from build123d import *

# Parameters (mm, degrees)
F1_DEPTH = 63.5
F2_DEPTH = 25.4
F0_W     = 25.4
F0_H     = 19.05
F3_DEPTH = 25.4
F4_DEPTH = 7.9375
F5_R     = 6.35


with BuildPart() as f1:
    # F0 (on Front) → F1 (new body, symmetric)
    with BuildSketch(Plane.XZ):
        Polygon((41.275, -9.525), (41.275, 9.525), (22.225, 9.525), (-41.275, 9.525), (-41.275, -9.525), align=None)
    extrude(amount=F1_DEPTH, both=True)

    # F0 (on Front) → F2 (join, symmetric)
    with BuildSketch(Plane.XZ):
        with BuildLine():
            Line((22.225, 9.525), (41.275, 9.525))
            Line((41.275, 9.525), (41.275, 27.0002))
            ThreePointArc((41.275, 27.0002), (45.9246798487, 38.2255201513), (57.15, 42.8752))
            Line((57.15, 42.8752), (60.325, 42.8752))
            Line((60.325, 42.8752), (60.325, 61.9252))
            Line((60.325, 61.9252), (57.15, 61.9252))
            add(Edge.make_bspline(
                [(55.2366570208, 61.872750002), (55.8711155645, 61.8932498519), (56.5088935827, 61.9107444376), (57.15, 61.9252)],
                knots=[110.2536827307, 110.2536827307, 110.2536827307, 110.2536827307, 111.5045361635, 111.5045361635, 111.5045361635, 111.5045361635], degree=3))
            ThreePointArc((55.2366570208, 61.872750002), (31.7868463263, 51.0099076352), (22.225, 27.0002))
            Line((22.225, 27.0002), (22.225, 9.525))
        make_face()
    extrude(amount=F2_DEPTH, both=True)

    # F0 (on Front) → F3 (join, symmetric)
    with BuildSketch(Plane.XZ):
        with Locations((73.025, 52.4002)):
            Rectangle(F0_W, F0_H)
    extrude(amount=F3_DEPTH, both=True)

    # F0 (on Front) → F4 (join, symmetric)
    with BuildSketch(Plane.XZ):
        with BuildLine():
            Line((-41.275, 9.525), (22.225, 9.525))
            Line((22.225, 9.525), (22.225, 27.0002))
            ThreePointArc((22.225, 27.0002), (31.7868463263, 51.0099076352), (55.2366570208, 61.872750002))
            add(Edge.make_bspline(
                [(-41.275, 9.525), (-30.8197184048, 34.9105826404), (-0.6862745856, 60.0658365111), (55.2366570208, 61.872750002)],
                knots=[0, 0, 0, 0, 110.2536827307, 110.2536827307, 110.2536827307, 110.2536827307], degree=3))
        make_face()
    extrude(amount=F4_DEPTH, both=True)

    # F5
    f5_edges = [f1.edges().sort_by_distance(p)[0] for p in [
        (-41.275, -63.5, 0),
        (41.275, -63.5, 0),
        (-41.275, 63.5, 0),
        (41.275, 63.5, 0),
    ]]
    fillet(f5_edges, radius=F5_R)


solid = f1.part
Geometry: final body of the model. Coordinates: model frame, mm. A direction names the side the tool comes from. Give positions to 0.01 mm unless a question says otherwise; leave off trailing zeros. Write each loop counter-clockwise with the first axis right and the second up, starting at its lowest first coordinate (ties: lowest second). Pieces come first, ordered by that corner, then holes. Notation, with made-up numbers: (16.5, -31.75) - (72.5, -31.75) arc R35 ccw to (72.5, 4.25) - close; hole circle Ø1 at (81.25, -18.75). An arc over 180 degrees is marked (long way). Return JSON: item names as keys, results as strings. Group by question number.
1) Section C-C on x = 72.5. Return the cut outline in (y, z).
2) Line query: line 1 (Z direction, x = 1, y = -45.5) (3 decimals); line 2 (Y direction, x = -10, z = 26); line 3 (X direction, y = 20.5, z = 15.5) (3 decimals). Output: solid intervals per line, ascending.
3) Set-up query: faces 1 (the flat face through (46, 25.4, 42)), 2 (the flat face through (46, -25.4, 42)), 3 (the flat face through (71, 0, 42.875)), 4 (the flat face through (-4, 7.938, 30)), 5 (the cylindrical face through (32.043, -16.791, 51.278)). Return all of +Z, -Z, +X, -X, +Y, -Y with unobstructed straight access to the full face (end or side cutting, diameter ignored); none if empty.
4) Section A-A on z = 3.5. Return the cut outline in (x, y) (3 decimals), plus the area to 3 significant figures.
5) Section B-B on y = -48. Return the cut outline in (x, z) (3 decimals).
6) First-contact query: P1, Ø2, axis at x = 0, z = 11, coming from the +Y side; P2, Ø15.5, axis at x = -3, z = 35, coming from the -Y side; P3, Ø15.5, axis at x = 44, z = 45.5, coming from the -Y side. Flat tips, straight axial feed; report the tip coordinate or a pass-through.
Filled in:
{
 "1": {"outline": "(-25.4, 42.88) - (25.4, 42.88) - (25.4, 61.93) - (-25.4, 61.93) - close"},
 "2": {"line 1": "z = -9.525 to 9.525", "line 2": "y = -7.94 to 7.94", "line 3": "x = 22.225 to 41.275"},
 "3": {"face 1": "+Z, +X, -X, +Y", "face 2": "+Z, +X, -X, -Y", "face 3": "-Z, +X, +Y, -Y", "face 4": "+Z, -X, +Y", "face 5": "+Z, -X, -Y"},
 "4": {"outline": "(-41.275, -57.15) arc R6.35 ccw to (-34.925, -63.5) - (34.925, -63.5) arc R6.35 ccw to (41.275, -57.15) - (41.275, 57.15) arc R6.35 ccw to (34.925, 63.5) - (-34.925, 63.5) arc R6.35 ccw to (-41.275, 57.15) - close", "area": "10,400 mm^2"},
 "5": {"outline": "(-41.275, -9.525) - (41.275, -9.525) - (41.275, 9.525) - (-41.275, 9.525) - close"},
 "6": {"P1": "stops at y = 7.94", "P2": "stops at y = -7.94", "P3": "stops at y = -25.4"}
}
